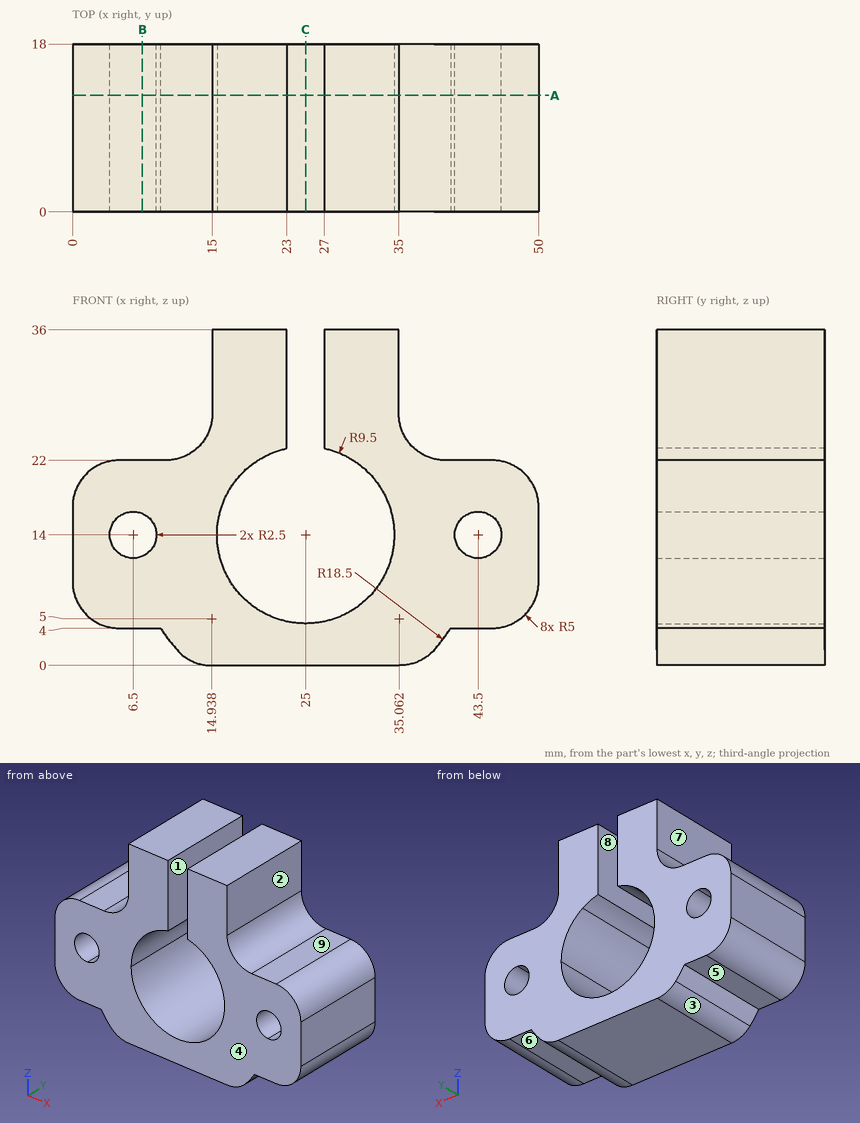
Job drawing, mm, ordinate dimensions from the low corner. One solid piece. A direction names the side the tool comes from. Round coordinates to 2 decimals unless told otherwise and drop trailing zeros. Write each loop counter-clockwise with the first axis right and the second up, starting at its lowest first coordinate (ties: lowest second). Pieces come first, ordered by that corner, then holes. Notation, with made-up numbers: M 82.5,-35 L 94.5,-35 A30 ccw 94.5,-13 Z; hole C -39,39 d11. An arc over 180 degrees is marked long. Return JSON: item names as keys, results as strings. Group by question number.
(1) Two-plate mould, pull along X, no slides. Class the marked faces 1, 2, 3 and 4: +X half, -X half, draft (parallel to the pull), parting line (faces both ways), or undercut.
(2) Pin check, flat tips, straight feed: pin 1 Ø4.5 at (y, z) = (5, 29.5) entering from -X; pin 2 Ø10 at (x, z) = (21.5, 16) entering from +Y; pin 3 Ø4 at (x, y) = (43, 11.5) entering from +Z; pin 4 Ø1 at (y, z) = (10, 18) entering from -X (3 decimals). Stop position of each tip, or through.
(3) Saw through at A-A on y = 12.5. Write the cut outline in (x, z) (1 decimal), then the cut area to 3 significant figures.
(4) Saw through at B-B on x = 7.5. Write the cut outline in (y, z).
(5) Drill centre lines: probe 1 along X at (y, z) = (13.75, 31.5); probe 2 along Z at (x, y) = (28, 4); probe 3 along X at (y, z) = (1, 13.5). Where is each one in solid material? Low to high.
(6) Saw through at C-C on x = 25. Write the cut outline in (y, z), then the cut area to 3 significant figures.
(7) Which spindle directions (+Z, -Z, +X, -X, +Y, -Y) get a long thin tool onto all of the face, cutting with end or side? Do the marked faces 5, 6, 7, 8 and 9. Say none if no direction does.
Returned:
{
 "1": {"face 1": "undercut", "face 2": "+X half", "face 3": "-X half", "face 4": "draft"},
 "2": {"pin 1": "x = 15", "pin 2": "through", "pin 3": "z = 22", "pin 4": "x = 0.025"},
 "3": {"outline": "M 0,9 A5 ccw 5,4 L 9.4,4 A18.5 ccw 11.2,1.7 A5 ccw 14.9,0 L 35.1,0 A5 ccw 38.8,1.7 A18.5 ccw 40.6,4 L 45,4 A5 ccw 50,9 L 50,17 A5 ccw 45,22 L 40,22 A5 cw 35,27 L 35,36 L 27,36 L 27,23.3 A9.5 cw long 23,23.3 L 23,36 L 15,36 L 15,27 A5 cw 10,22 L 5,22 A5 ccw 0,17 Z; hole C 6.5,14 d5; hole C 43.5,14 d5", "area": "907 mm²"},
 "4": {"outline": "M 0,4 L 18,4 L 18,11.71 L 0,11.71 Z; M 0,16.29 L 18,16.29 L 18,22 L 0,22 Z"},
 "5": {"probe 1": "15 to 23, 27 to 35", "probe 2": "0 to 4.99, 23.01 to 36", "probe 3": "0 to 4.05, 8.95 to 15.51, 34.49 to 41.05, 45.95 to 50"},
 "6": {"outline": "M 0,0 L 18,0 L 18,4.5 L 0,4.5 Z", "area": "81.0 mm²"},
 "7": {"face 5": "-Z, -X, +Y, -Y", "face 6": "-Z, +X, +Y, -Y", "face 7": "+Z, -X, +Y, -Y", "face 8": "+Z, +Y, -Y", "face 9": "+Z, +X, +Y, -Y"}
}
